Verification items for the finished model (mm, model axes). A direction names the side the tool comes from. Round coordinates to 2 decimals unless told otherwise and drop trailing zeros. Order: outer loops, then holes, each group sorted by start corner. A loop starts at its lowest first (then second) coordinate and runs counter-clockwise, first axis right, second up. Notation, with made-up numbers: (4.5, -14) -> (33.5, -14) arc R25 cw to (33.5, 22) -> close; hole circle Ø9 at (13, 35). An arc over 180 degrees is marked (long way). Answer in a Markdown table with one row per item. Add a question column.
```python
from build123d import *

# Parameters (mm, degrees)
ESQUISSE1_W        = 120
ESQUISSE1_H        = 40
BOSS_EXTRU_1_DEPTH = 6
ESQUISSE2_W        = 50
ESQUISSE2_H        = 6
BOSS_EXTRU_2_DEPTH = 6
CUT_EXTRUDE1_DEPTH = 40
CUT_EXTRUDE2_DEPTH = 40
SKETCH3_W          = 1
SKETCH3_H          = 40
SKETCH3_H_2        = 6
CUT_EXTRUDE3_DEPTH = 7


with BuildPart() as part:
    # Esquisse1 → Boss.-Extru.1 (new body)
    with BuildSketch(Plane.XY):
        Rectangle(ESQUISSE1_W, ESQUISSE1_H)
    extrude(amount=BOSS_EXTRU_1_DEPTH)

    # Esquisse2 → Boss.-Extru.2 (add)
    with BuildSketch(Plane.XY.offset(6)):
        with Locations((0, 23)):
            Rectangle(ESQUISSE2_W, ESQUISSE2_H)
    extrude(amount=-BOSS_EXTRU_2_DEPTH)

    # Sketch1 → Cut-Extrude1 (cut)
    with BuildSketch(Plane.ZY.offset(60)):
        Polygon((6, -20), (0, -14), (0, -20), align=None)
    extrude(amount=-CUT_EXTRUDE1_DEPTH, mode=Mode.SUBTRACT)

    # Sketch2 → Cut-Extrude2 (cut)
    with BuildSketch(Plane(origin=(60, 0, 0), x_dir=(0, 0, -1), z_dir=(1, 0, 0))):
        Polygon((-6, -20), (0, -14), (0, -20), align=None)
    extrude(amount=-CUT_EXTRUDE2_DEPTH, mode=Mode.SUBTRACT)

    # Sketch3 → Cut-Extrude3 (cut, through all)
    with BuildSketch(Plane.XY.offset(6)):
        with Locations((59.5, 0)):
            Rectangle(SKETCH3_W, SKETCH3_H)
        with Locations((24.5, 23)):
            Rectangle(SKETCH3_W, SKETCH3_H_2)
        with Locations((-24.5, 23)):
            Rectangle(SKETCH3_W, SKETCH3_H_2)
        with Locations((-59.5, 0)):
            Rectangle(SKETCH3_W, SKETCH3_H)
    extrude(amount=-CUT_EXTRUDE3_DEPTH, mode=Mode.SUBTRACT)


solid = part.part
```
1) Cross-section at C-C, the plane y = 21.5. Record the boundary of the cut face in (x, z), and give its area (3 significant figures).
2) Tool access check on faces 1 (the face through (41, 20, 3)), 2 (the face through (20, -18, 2)), 3 (the face through (-20, -18, 2)), 4 (the face through (-24, 23, 3)), 5 (the face through (0, -20, 3)). Record the directions out of +Z, -Z, +X, -X, +Y, -Y that give a thin tool (end or side, any length) a straight path to the whole face; none if there is none.
3) Depth check by flat-ended pin: P1, Ø1.8, axis at x = 39.5, z = 2, coming from the +Y side. Enter the tip coordinate at first touch or a pass-through.
4) Cross-section at A-A, the plane z = 3. Record the boundary of the cut face in (x, y).
5) Thickness scan on L1, parallel to X at y = 23.5, z = 2.75; L2, parallel to Y at x = 49.5, z = 3.5; L3, parallel to Y at x = 34.5, z = 2.5. Record the ranges inside material, lowest first. Write a range as [from, to].
6) Cross-section at B-B, the plane x = 29. Record the boundary of the cut face in (y, z), and give its area (3 significant figures).
Results below:
| question | item | result |
|---|---|---|
| 1 | outline | (-24, 0) -> (24, 0) -> (24, 6) -> (-24, 6) -> close |
| 1 | area | 288 mm² |
| 2 | face 1 | +Z, -Z, +X, +Y |
| 2 | face 2 | -Z, +X, -Y |
| 2 | face 3 | -Z, -X, -Y |
| 2 | face 4 | +Z, -Z, -X, +Y |
| 2 | face 5 | +Z, -Z, +X, -X, -Y |
| 3 | P1 | y = 20 |
| 4 | outline | (-59, -17) -> (-20, -17) -> (-20, -20) -> (20, -20) -> (20, -17) -> (59, -17) -> (59, 20) -> (24, 20) -> (24, 26) -> (-24, 26) -> (-24, 20) -> (-59, 20) -> close |
| 5 | L1 | [-24, 24] |
| 5 | L2 | [-17.5, 20] |
| 5 | L3 | [-16.5, 20] |
| 6 | outline | (-20, 6) -> (-14, 0) -> (20, 0) -> (20, 6) -> close |
| 6 | area | 222 mm² |
